from build123d import *

# Parameters (mm, degrees)
SKETCH1_W           = 40
SKETCH1_H           = 60
BOSS_EXTRUDE1_DEPTH = 3
SKETCH2_R           = 2.15
SKETCH2_W           = 20
SKETCH2_H           = 40
CUT_EXTRUDE1_DEPTH  = 3
SKETCH3_W           = 5
SKETCH3_H           = 3
BOSS_EXTRUDE2_DEPTH = 3
SKETCH4_W           = 3
SKETCH4_H           = 5
CUT_EXTRUDE2_DEPTH  = 3


with BuildPart() as part:
    # Sketch1 → Boss-Extrude1 (new body)
    with BuildSketch(Plane.XY):
        Rectangle(SKETCH1_W, SKETCH1_H)
    extrude(amount=BOSS_EXTRUDE1_DEPTH)

    # Sketch2 → Cut-Extrude1 (cut)
    with BuildSketch(Plane.XY.offset(3)):
        with Locations((4.845, 24.49)):
            Circle(SKETCH2_R)
        with Locations((-5.025, 24.49)):
            Circle(SKETCH2_R)
        with Locations((-5.025, -24.81)):
            Circle(SKETCH2_R)
        with Locations((4.845, -24.81)):
            Circle(SKETCH2_R)
        Rectangle(SKETCH2_W, SKETCH2_H)
    extrude(amount=-CUT_EXTRUDE1_DEPTH, mode=Mode.SUBTRACT)

    # Sketch3 → Boss-Extrude2 (add)
    with BuildSketch(Plane.XZ.offset(30)):
        with Locations((12.5, 1.5)):
            Rectangle(SKETCH3_W, SKETCH3_H)
        with Locations((-12.5, 1.5)):
            Rectangle(SKETCH3_W, SKETCH3_H)
    extrude(amount=BOSS_EXTRUDE2_DEPTH)

    # Sketch4 → Cut-Extrude2 (cut)
    with BuildSketch(Plane(origin=(0, 0, 0), x_dir=(-1, 0, 0), z_dir=(0, 0, -1))):
        with Locations((-18.5, -22.5)):
            Rectangle(SKETCH4_W, SKETCH4_H)
        with Locations((-18.5, 22.5)):
            Rectangle(SKETCH4_W, SKETCH4_H)
        with Locations((18.5, 22.5)):
            Rectangle(SKETCH4_W, SKETCH4_H)
        with Locations((18.5, -22.5)):
            Rectangle(SKETCH4_W, SKETCH4_H)
    extrude(amount=-CUT_EXTRUDE2_DEPTH, mode=Mode.SUBTRACT)


solid = part.part
Geometry: final body of the model. Coordinates: model frame, mm. A direction names the side the tool comes from. Give positions to 0.01 mm unless a question says otherwise; leave off trailing zeros. Loops run counter-clockwise (first coordinate to the right, second up) from the corner with the lowest first, then second, coordinate; pieces in that order, holes last. Notation, with made-up numbers: (54.5, 17) - (59.5, 17) arc R20 ccw to (59.5, 25) - close; hole circle Ø7 at (15, -16). An arc over 180 degrees is marked (long way). Answer as CSV lines item,"result". Start each with the question number.
1. Draft query along Y for faces 1 (the face through (0, 30, 1)), 2 (the face through (-13, -33, 2)), 3 (the face through (-15, -31, 1)), 4 (the face through (-10, 0, 2)). Return one class per face: released by +Y, released by -Y, zero draft, split by the parting line, or undercut.
2. Pin query (flat end, axial travel): P1, Ø1.5, axis at x = 4, z = 1.5, coming from the -Y side; P2, Ø1.5, axis at y = -31, z = 2, coming from the +X side. Return the tip coordinate at first contact, or that it passes through.
3. Section D-D, the plane z = 1. Give the number of separate pieces and of enclosed holes in the cut face, plus the area to 3 significant figures.
4. Reachability of faces 5 (the face through (-18, -30, 1)), 6 (the face through (17, -30, 1)), 7 (the face through (0, 20, 2)) from +Z, -Z, +X, -X, +Y, -Y: full face, straight path, thin tool, end or side. Return the list, or none.
5. Ray query, L1, parallel to Y at x = 5, z = 0.85; L2, parallel to Y at x = 18, z = 1.05; L3, parallel to Y at x = 9.5, z = 0.25. Return the intervals inside material, ascending.
6. Section C-C, the plane y = -26. Return loops of the section in (x, z), plus the area to 3 significant figures.
7. Section B-B, the plane y = -3.5. Return loops of the section in (x, z), plus the area to 3 significant figures.
8. Section A-A, the plane x = -2. Return loops of the section in (y, z), plus the area to 3 significant figures.
Answers:
1,face 1,"released by +Y"
1,face 2,"released by -Y"
1,face 3,"zero draft"
1,face 4,"undercut"
2,P1,"stops at y = -30"
2,P2,"stops at x = 15"
3,separate pieces,"1"
3,enclosed holes,"5"
3,area,"1,510 mm2"
4,face 5,"+Z, -Z, -X, -Y"
4,face 6,"+Z, -Z, +X, -Y"
4,face 7,"+Z, -Z"
5,L1,"y = -30 to -26.95, -22.67 to -20, 20 to 22.35, 26.63 to 30"
5,L2,"y = -30 to -25, -20 to 20, 25 to 30"
5,L3,"y = -30 to -20, 20 to 30"
6,outline,"(-20, 0) - (-6.82, 0) - (-6.82, 3) - (-20, 3) - close; (-3.23, 0) - (3.05, 0) - (3.05, 3) - (-3.23, 3) - close; (6.64, 0) - (20, 0) - (20, 3) - (6.64, 3) - close"
6,area,"98.5 mm2"
7,outline,"(-20, 0) - (-10, 0) - (-10, 3) - (-20, 3) - close; (10, 0) - (20, 0) - (20, 3) - (10, 3) - close"
7,area,"60.0 mm2"
8,outline,"(-30, 0) - (-20, 0) - (-20, 3) - (-30, 3) - close; (20, 0) - (30, 0) - (30, 3) - (20, 3) - close"
8,area,"60.0 mm2"
